For this review, take the finished solid that the model builds, in its own axes (mm). Face numbers are marked on the shaded views. A direction names the side the tool comes from. Coordinates: 2 decimals unless noted, no trailing zeros. Order: outer loops, then holes, each group sorted by start corner. A loop starts at its lowest first (then second) coordinate and runs counter-clockwise, first axis right, second up. Notation, with made-up numbers: (68.25, 0.5) -> (90.25, 0.5) arc R32 cw to (90.25, 27.5) -> close; hole circle Ø11 at (49.5, -19). An arc over 180 degrees is marked (long way). Write item = value, one per line. Start each with the question number.
1) Consider section D-D on x = 95. Give the boundary of the cut face in (y, z).
2) Machinability: for the marked faces 4 and 5, which of the approach directions +Z, -Z, +X, -X, +Y, -Y give a long, thin tool a straight path to every point of the face, cutting with its end or side? Answer none if there is none.
3) Consider section C-C on x = -3.5. Give the boundary of the cut face in (y, z).
4) Wall thickness on probe 1 along Z at (x, y) = (16, -39); probe 2 along X at (y, z) = (-31.5, 36.5); probe 3 along Y at (x, z) = (40, 11.5): over which ranges is each line inside the solid? List them lowest first. Write a range as [from, to].
5) Draft analysis for pull direction X (two halves, no side actions). For the marked faces 1, 2 and 3, state which applies: +X half, -X half, draft (parallel to the pull), parting line (faces both ways), or undercut.
6) Consider section B-B on y = -29. Give the boundary of the cut face in (x, z), and give its area (3 significant figures).
7) Insertion check: pin 1 Ø5 at (x, z) = (31, 19) entering from +Y; pin 2 Ø8 at (x, z) = (94, 21.5) entering from -Y; pin 3 Ø8 at (x, y) = (51, -36) entering from -Z. Each pin has a flat end and moves straight along its axis. Give the tip position at first contact, or say it passes through.
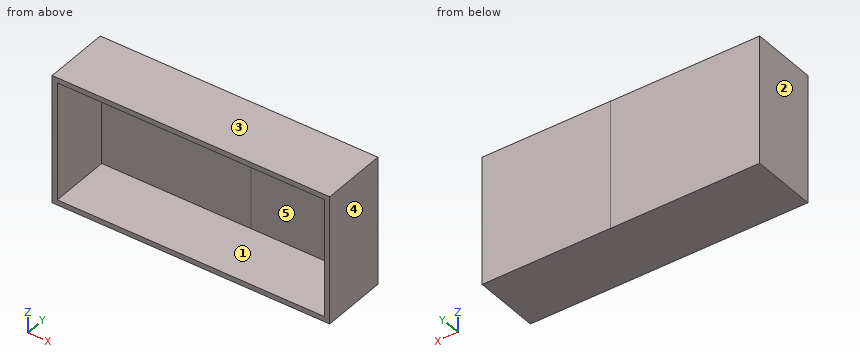
from build123d import *

# Parameters (mm, degrees)
F0_W     = 73.8667733967
F0_H     = 32.6388925314
F1_DEPTH = 63.5
F2_T     = -2.54


with BuildPart() as f1:
    # F0 (on Top) → F1 (new body)
    with BuildSketch(Plane.XY):
        Polygon((46.6460995376, -18.4034332633), (46.6460995376, -51.0423257947), (110.020622611, -51.0423257947), (110.020622611, -18.363982439), (46.6460995376, -18.363982439), align=None)
        with Locations((9.7127128392, -34.722879529)):
            Rectangle(F0_W, F0_H)
    extrude(amount=F1_DEPTH)

    # F2
    f2_openings = [f1.faces().sort_by_distance(p)[0] for p in [
        (41.399974, -51.042326, 31.75),
    ]]
    offset(amount=F2_T, openings=f2_openings, kind=Kind.INTERSECTION)


solid = f1.part
Answer sheet:
q1.outline = (-51.04, 0) -> (-18.36, 0) -> (-18.36, 63.5) -> (-51.04, 63.5) -> (-51.04, 60.96) -> (-20.9, 60.96) -> (-20.9, 2.54) -> (-51.04, 2.54) -> close
q2.face_4 = +Z, -Z, +X, +Y, -Y
q2.face_5 = -Y
q3.outline = (-51.04, 0) -> (-18.4, 0) -> (-18.4, 63.5) -> (-51.04, 63.5) -> (-51.04, 60.96) -> (-20.94, 60.96) -> (-20.94, 2.54) -> (-51.04, 2.54) -> close
q4.probe_1 = [0, 2.54], [60.96, 63.5]
q4.probe_2 = [-27.22, -24.68], [107.48, 110.02]
q4.probe_3 = [-20.94, -18.4]
q5.face_1 = undercut
q5.face_2 = -X half
q5.face_3 = draft
q6.outline = (-27.22, 0) -> (110.02, 0) -> (110.02, 63.5) -> (-27.22, 63.5) -> close; hole (-24.68, 2.54) -> (107.48, 2.54) -> (107.48, 60.96) -> (-24.68, 60.96) -> close
q6.area = 994 mm2
q7.pin_1 = -18.4
q7.pin_2 = -20.9
q7.pin_3 = 0
